For this review, take the finished solid that the model builds, in its own axes (mm). Give positions to 0.01 mm unless a question says otherwise; leave off trailing zeros. Write each loop counter-clockwise with the first axis right and the second up, starting at its lowest first coordinate (ties: lowest second). Pieces come first, ordered by that corner, then holes.
Q1. We need section D-D (y = 35). Write out the cut boundary in (x, z).
Q2. We need section C-C (z = 0.5). Give the number of separate pieces and of enclosed holes in the cut face, then the cut area to 3 significant figures.
Q3. We need section A-A (y = 0). Write out the cut boundary in (x, z), then the cut area to 3 significant figures.
Q4. For line 1 (Y direction, x = 1, z = 0.95); line 2 (Y direction, x = 25, z = 0.75); line 3 (X direction, y = -32.5, z = 0.65), list the stretches that pass through material, from the lowest coordinate up.
Q5. Mouldability with a two-part tool opening along X and no side actions: class faces 1 (the flat face through (6, 30, 0)), 2 (the cylindrical face through (24.467, -24.441, 0.493)), 3 (the cylindrical face through (-8.67, -39.05, 0.49)) as released by +X, released by -X, zero draft, split by the parting line, or undercut.
Q6. Insertion check: P1, Ø4.5, axis at x = -26.45, y = -22.92, coming from the -Z side. The pin has a flat end and moves straight along its axis. Give the tip position at first contact, or say it passes through.
Q7. We need section B-B (x = 0). Write out the cut boundary in (y, z), then the cut area to 3 significant figures.
```python
from build123d import *

# Parameters (mm, degrees)
SKETCH1_R           = 40
SKETCH1_R_2         = 30
SKETCH1_R_3         = 2.5
BOSS_EXTRUDE1_DEPTH = 1


with BuildPart() as part:
    # Sketch1 → Boss-Extrude1 (new body)
    with BuildSketch(Plane.XY):
        Circle(SKETCH1_R)
        Circle(SKETCH1_R_2, mode=Mode.SUBTRACT)
        with Locations((0, 35)):
            Circle(SKETCH1_R_3, mode=Mode.SUBTRACT)
        with Locations((18.922428611, 29.443873649)):
            Circle(SKETCH1_R_3, mode=Mode.SUBTRACT)
        with Locations((31.837119837, 14.539525455)):
            Circle(SKETCH1_R_3, mode=Mode.SUBTRACT)
        with Locations((34.643750466, -4.98101934)):
            Circle(SKETCH1_R_3, mode=Mode.SUBTRACT)
        with Locations((26.451235102, -22.920125688)):
            Circle(SKETCH1_R_3, mode=Mode.SUBTRACT)
        with Locations((9.860639489, -33.582254077)):
            Circle(SKETCH1_R_3, mode=Mode.SUBTRACT)
        with Locations((-9.860639489, -33.582254077)):
            Circle(SKETCH1_R_3, mode=Mode.SUBTRACT)
        with Locations((-26.451235102, -22.920125688)):
            Circle(SKETCH1_R_3, mode=Mode.SUBTRACT)
        with Locations((-34.643750466, -4.98101934)):
            Circle(SKETCH1_R_3, mode=Mode.SUBTRACT)
        with Locations((-31.837119837, 14.539525455)):
            Circle(SKETCH1_R_3, mode=Mode.SUBTRACT)
        with Locations((-18.922428611, 29.443873649)):
            Circle(SKETCH1_R_3, mode=Mode.SUBTRACT)
    extrude(amount=BOSS_EXTRUDE1_DEPTH)


solid = part.part
```
Computed:
1. outline: (-19.36, 0) - (-2.5, 0) - (-2.5, 1) - (-19.36, 1) - close; (2.5, 0) - (19.36, 0) - (19.36, 1) - (2.5, 1) - close
2. separate pieces: 1
2. enclosed holes: 12
2. area: 1,980 mm2
3. outline: (-40, 0) - (-30, 0) - (-30, 1) - (-40, 1) - close; (30, 0) - (40, 0) - (40, 1) - (30, 1) - close
3. area: 20.0 mm2
4. line 1: y = -39.99 to -29.98, 29.98 to 32.71, 37.29 to 39.99
4. line 2: y = -31.22 to -24.96, -20.88 to -16.58, 16.58 to 31.22
4. line 3: x = -23.32 to -12.11, -7.61 to 7.61, 12.11 to 23.32
5. face 1: zero draft
5. face 2: undercut
5. face 3: split by the parting line
6. P1: passes through
7. outline: (-40, 0) - (-30, 0) - (-30, 1) - (-40, 1) - close; (30, 0) - (32.5, 0) - (32.5, 1) - (30, 1) - close; (37.5, 0) - (40, 0) - (40, 1) - (37.5, 1) - close
7. area: 15.0 mm2
